Study the drawing (mm; zero at the part's minimum x, y, z) and answer. A direction names the side the tool comes from. Coordinates: 2 decimals unless noted, no trailing zeros. Order: outer loops, then holes, each group sorted by start corner. A loop starts at its lowest first (then second) coordinate and runs counter-clockwise, first axis right, second up.
1. Determine the mould class of the marked faces 1, 2, 3 and 4 for opening direction Z: +Z half, -Z half, draft (parallel to the pull), parting line (faces both ways), or undercut.
2. Find the intervals of material crossed by probe 1 along X at (y, z) = (61.5, 36.5); probe 2 along Y at (x, z) = (55.5, 8); probe 3 along Y at (x, z) = (92, 14.5), in increasing order.
3. The part is cut by section A-A, the plane y = 44.5. Give the vertices of the cut face in (x, z) (1 decimal).
4. The part is cut by section D-D, the plane y = 57. Give the vertices of the cut face in (x, z), then the cut area to 3 significant figures.
5. Flat-ended cylindrical pins translate along their axes: pin 1 Ø2 at (x, y) = (13, 39) entering from -Z; pin 2 Ø4 at (y, z) = (63, 53) entering from +X; pin 3 Ø21 at (x, z) = (57, 28) entering from +Y; pin 4 Ø9 at (x, z) = (96, 63.5) entering from +Y. Find the tip coordinate at first contact, or state that the pin passes through.
6. A tool of negligible diameter and unlimited length cuts with its end or side. For the marked faces 5, 6 and 7, from which of +Z, -Z, +X, -X, +Y, -Y can it reach the whole face along a straight path? Write none if from no direction.
7. The part is cut by section C-C, the plane z = 54.5. Give the vertices of the cut face in (x, y) (1 decimal), then the cut area to 3 significant figures.
8. The part is cut by section B-B, the plane x = 80. Give the vertices of the cut face in (y, z), then the cut area to 3 significant figures.
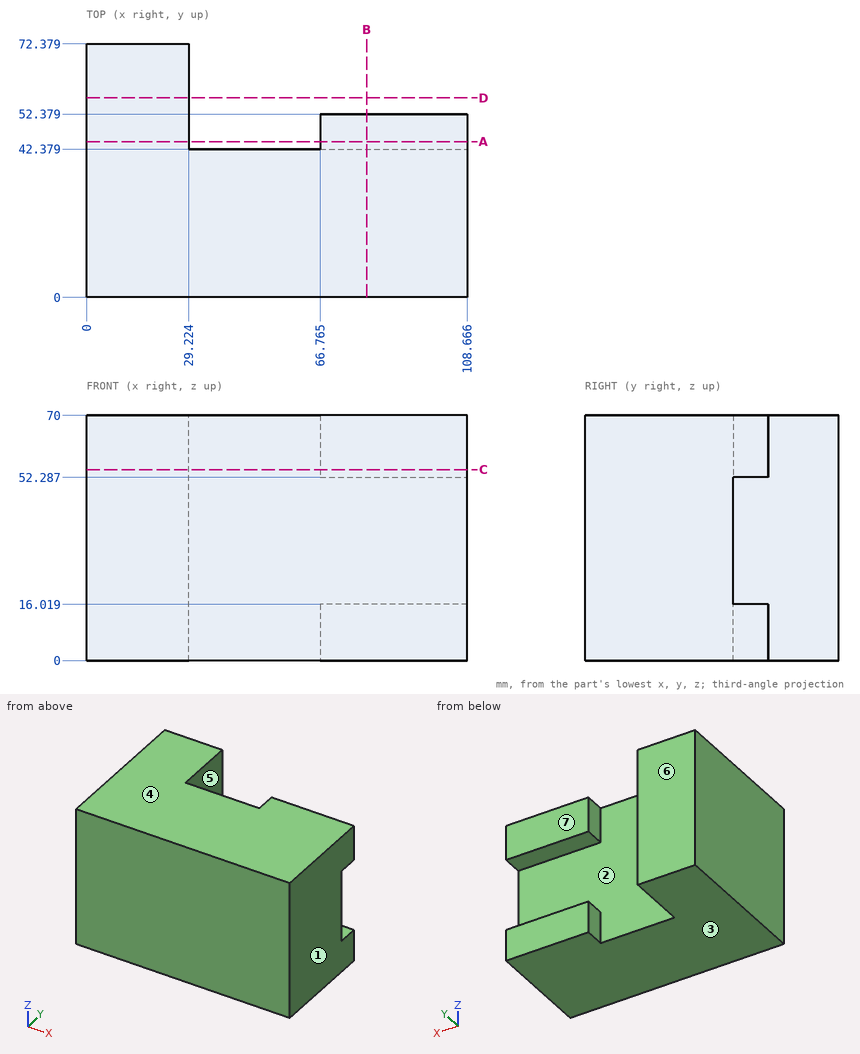
Geometry says:
1. face 1: draft
1. face 2: undercut
1. face 3: -Z half
1. face 4: +Z half
2. probe 1: x = 0 to 29.22
2. probe 2: y = 0 to 42.38
2. probe 3: y = 0 to 52.38
3. outline: (0, 0) - (29.2, 0) - (29.2, 70) - (0, 70) - close; (66.8, 0) - (108.7, 0) - (108.7, 16) - (66.8, 16) - close; (66.8, 52.3) - (108.7, 52.3) - (108.7, 70) - (66.8, 70) - close
4. outline: (0, 0) - (29.22, 0) - (29.22, 70) - (0, 70) - close
4. area: 2,050 mm2
5. pin 1: stops at z = 0
5. pin 2: stops at x = 29.22
5. pin 3: stops at y = 42.38
5. pin 4: stops at y = 52.38
6. face 5: +Z, -Z, +Y
6. face 6: +Z, -Z, +X, -X, +Y
6. face 7: +Z, -Z, +X, +Y
7. outline: (0, 0) - (108.7, 0) - (108.7, 52.4) - (66.8, 52.4) - (66.8, 42.4) - (29.2, 42.4) - (29.2, 72.4) - (0, 72.4) - close
7. area: 5,900 mm2
8. outline: (0, 0) - (52.38, 0) - (52.38, 16.02) - (42.38, 16.02) - (42.38, 52.29) - (52.38, 52.29) - (52.38, 70) - (0, 70) - close
8. area: 3,300 mm2
